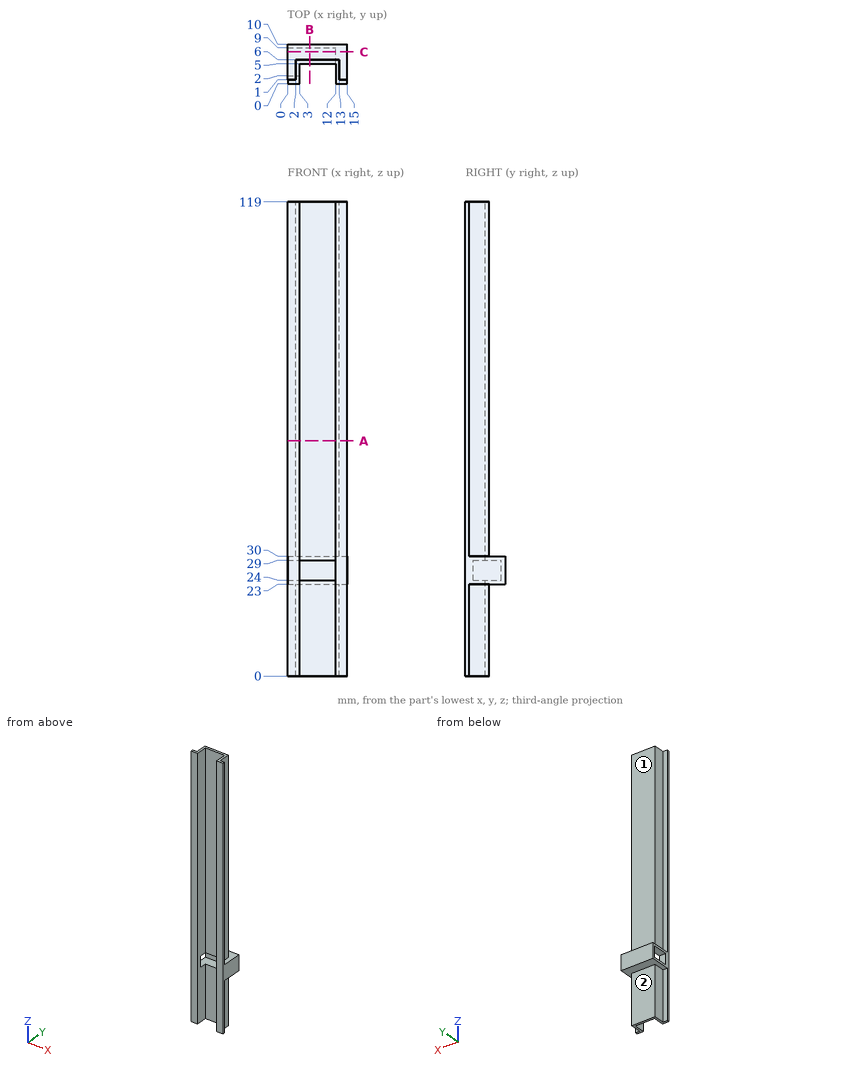
Here's the drawing with two shaded views (mm, measured from the low corner). I have some questions. A direction names the side the tool comes from. Coordinates: 2 decimals unless noted, no trailing zeros. Write each loop counter-clockwise with the first axis right and the second up, starting at its lowest first coordinate (ties: lowest second). Pieces come first, ordered by that corner, then holes.
Item 1: Will these pins go through, and if not, where does the flat tip stop? pin 1 (1 mm diameter, centred on x = 14, z = 71, fed in from +Y); pin 2 (5.5 mm diameter, centred on y = 2.5, z = 63.5, fed in from -X); pin 3 (4.5 mm diameter, centred on y = 3.5, z = 59.5, fed in from -X); pin 4 (2 mm diameter, centred on x = 8.5, z = 93.5, fed in from -Y).
Item 2: On a 3-axis mill with a long thin cutter (end or side, diameter ignored), from which of +Z, -Z, +X, -X, +Y, -Y can I reach the whole of each face in a straight line? I mean the marked faces 1 and 2. Say none if no direction works.
Item 3: I want a section at A-A on z = 59. Write out the boundary of the cut face in (x, y), and give its area (3 significant figures).
Item 4: If I drill on line 1 (X direction, y = 4.5, z = 54); line 2 (Z direction, x = 0.5, y = 8.75); line 3 (Y direction, x = 14, z = 96), over which ranges is the centre line in solid material (lowest first)?
Item 5: I want a section at C-C on y = 8. Write out the boundary of the cut face in (x, z), and give its area (3 significant figures).
Item 6: I want a section at B-B on x = 5.5. Write out the boundary of the cut face in (y, z).
Findings below:
1. pin 1: stops at y = 1
1. pin 2: stops at x = 0
1. pin 3: stops at x = 2
1. pin 4: stops at y = 5
2. face 1: +Z, +X, -X, +Y
2. face 2: -Z, +X, -X, +Y
3. outline: (0, 0) - (3, 0) - (3, 5) - (12, 5) - (12, 0) - (15, 0) - (15, 1) - (13, 1) - (13, 6) - (2, 6) - (2, 1) - (0, 1) - close
3. area: 25.0 mm2
4. line 1: x = 2 to 3, 12 to 13
4. line 2: z = 23 to 24, 29 to 30
4. line 3: y = 0 to 1
5. outline: (0, 23) - (15, 23) - (15, 30) - (0, 30) - (0, 29) - (12, 29) - (12, 24) - (0, 24) - close
5. area: 45.0 mm2
6. outline: (5, 0) - (6, 0) - (6, 23) - (10, 23) - (10, 30) - (6, 30) - (6, 119) - (5, 119) - (5, 29) - (9, 29) - (9, 24) - (5, 24) - close
